```python
from build123d import *

# Parameters (mm, degrees)
SKETCH1_W             = 10
SKETCH1_H             = 15
BOSS_EXTRUDE1_DEPTH   = 1.6
FILLET1_R             = 1.5
SKETCH2_R             = 3.45
BOSS_EXTRUDE2_DEPTH   = 1.4
M5X0_8_TAPPED_HOLE1_D = 4.2
FILLET2_R             = 0.4


with BuildPart() as part:
    # Sketch1 → Boss-Extrude1 (new body)
    with BuildSketch(Plane(origin=(0, 0, 0), x_dir=(1, 0, 0), z_dir=(0, 1, 0))):
        with Locations((5, 7.5)):
            Rectangle(SKETCH1_W, SKETCH1_H)
    extrude(amount=BOSS_EXTRUDE1_DEPTH)

    # Fillet1
    fillet1_edges = [part.edges().sort_by_distance(p)[0] for p in [
        (0, 0.8, -15),
        (10, 0.8, -15),
        (10, 0.8, 0),
        (0, 0.8, 0),
    ]]
    fillet(fillet1_edges, radius=FILLET1_R)

    # Sketch2 → Boss-Extrude2 (add)
    with BuildSketch(Plane.XZ):
        with Locations(Location((5, -7.5, 0), (0, 0, 270))):
            Circle(SKETCH2_R)
    extrude(amount=BOSS_EXTRUDE2_DEPTH)

    # M5x0.8 Tapped Hole1 (through all)
    with Locations(Plane(origin=(0, 1.6, 0), x_dir=(1, 0, 0), z_dir=(0, 1, 0))):
        with Locations((5, 7.5)):
            Hole(M5X0_8_TAPPED_HOLE1_D / 2)

    # Fillet2
    fillet2_edges = [part.edges().sort_by_distance(p)[0] for p in [
        (5, 0, -4.05),
    ]]
    fillet(fillet2_edges, radius=FILLET2_R)


solid = part.part
```
Here's how the part is built. I have some questions about the finished solid (model axes, mm). A direction names the side the tool comes from. Coordinates: 2 decimals unless noted, no trailing zeros. Order: outer loops, then holes, each group sorted by start corner. A loop starts at its lowest first (then second) coordinate and runs counter-clockwise, first axis right, second up. Notation, with made-up numbers: M -26.5,37.25 L -9.5,37.25 A25 ccw -9.5,53.25 Z; hole C -18,-5.75 d8. An arc over 180 degrees is marked long. Answer as a JSON object with one key per item and string values. Group by question number.
(1) Suppose I cut it at D-D, the plane z = -12.25. Please give me the cut outline in (x, y), then the cut area to 3 significant figures.
(2) Suppose I cut it at A-A, the plane z = -7.5. Please give me the cut outline in (x, y), then the cut area to 3 significant figures.
(3) I need wall thicknesses on probe 1 along Z at (x, y) = (5, 0.3); probe 2 along Y at (x, z) = (8.75, -3.5); probe 3 along Z at (x, y) = (6.25, 0.5). Which ranges of each line are inside material? Lowest first, please.
(4) Which directions (+Z, -Z, +X, -X, +Y, -Y) give clear straight access to the entire face, cutting with the end or side of a thin tool? Please do faces 1 (the face through (9.55, 0.81, -0.43)), 2 (the face through (6, -0.9, -10.8)).
(5) Suppose I cut it at B-B, the plane x = 5. Please give me the cut outline in (y, z), then the cut area to 3 significant figures.
(6) Suppose I cut it at C-C, the plane y = 0.5. Please give me the cut outline in (x, z), then the cut area to 3 significant figures.
(7) If we mould it in two halves opening along X, with no side actions, what happens to faces 3 (the face through (5.273, 0.079, -9.582)), 4 (the face through (0, 1, -7)), 5 (the face through (10, 1, -7)), 6 (the face through (3, 0, -4))? For each: released by +X, released by -X, zero draft, split by the parting line, or undercut.
Values found:
{
 "1": {"outline": "M 0,0 L 10,0 L 10,1.6 L 0,1.6 Z", "area": "16.0 mm^2"},
 "2": {"outline": "M 0,0 L 1.15,0 A0.4 cw 1.55,-0.4 L 1.55,-1.4 L 2.9,-1.4 L 2.9,1.6 L 0,1.6 Z; M 7.1,-1.4 L 8.45,-1.4 L 8.45,-0.4 A0.4 cw 8.85,0 L 10,0 L 10,1.6 L 7.1,1.6 Z", "area": "13.1 mm^2"},
 "3": {"probe 1": "z = -15 to -9.6, -5.4 to 0", "probe 2": "y = 0 to 1.6", "probe 3": "z = -15 to -9.19, -5.81 to 0"},
 "4": {"face 1": "+Z, +X, +Y, -Y", "face 2": "-Y"},
 "5": {"outline": "M -1.4,-10.95 L -0.4,-10.95 A0.4 cw 0,-11.35 L 0,-15 L 1.6,-15 L 1.6,-9.6 L -1.4,-9.6 Z; M -1.4,-5.4 L 1.6,-5.4 L 1.6,0 L 0,0 L 0,-3.65 A0.4 cw -0.4,-4.05 L -1.4,-4.05 Z", "area": "21.1 mm^2"},
 "6": {"outline": "M 0,-13.5 A1.5 ccw 1.5,-15 L 8.5,-15 A1.5 ccw 10,-13.5 L 10,-1.5 A1.5 ccw 8.5,0 L 1.5,0 A1.5 ccw 0,-1.5 Z; hole C 5,-7.5 d4.2", "area": "134 mm^2"},
 "7": {"face 3": "undercut", "face 4": "released by -X", "face 5": "released by +X", "face 6": "zero draft"}
}
